```python
from build123d import *

# Parameters (mm, degrees)
F0_W     = 70
F0_H     = 60
F1_DEPTH = 2
F2_R     = 7
F3_W     = 64
F3_H     = 54
F4_DEPTH = 3
F5_R     = 5
F6_T     = -2


with BuildPart() as f1:
    # F0 (on Front) → F1 (new body)
    with BuildSketch(Plane.XZ):
        Rectangle(F0_W, F0_H)
    extrude(amount=F1_DEPTH)

    # F2
    f2_edges = [f1.edges().sort_by_distance(p)[0] for p in [
        (-35, -1, 30),
        (35, -1, 30),
        (35, -1, -30),
        (-35, -1, -30),
    ]]
    fillet(f2_edges, radius=F2_R)

    # F3 (on face) → F4 (join)
    with BuildSketch(Plane(origin=(0, 0, 0), x_dir=(-1, 0, 0), z_dir=(0, 1, 0))):
        Rectangle(F3_W, F3_H)
    extrude(amount=F4_DEPTH)

    # F5
    f5_edges = [f1.edges().sort_by_distance(p)[0] for p in [
        (32, 1.5, 27),
        (-32, 1.5, 27),
        (32, 1.5, -27),
        (-32, 1.5, -27),
    ]]
    fillet(f5_edges, radius=F5_R)

    # F6
    f6_openings = [f1.faces().sort_by_distance(p)[0] for p in [
        (0, 3, 0),
    ]]
    offset(amount=F6_T, openings=f6_openings, kind=Kind.INTERSECTION)


solid = f1.part
```
Verification items for the finished model (mm, model axes). A direction names the side the tool comes from. Give positions to 0.01 mm unless a question says otherwise; leave off trailing zeros. Order: outer loops, then holes, each group sorted by start corner. A loop starts at its lowest first (then second) coordinate and runs counter-clockwise, first axis right, second up. Notation, with made-up numbers: M 0,45 L 14,45 A8 ccw 14,50 Z; hole C 25.5,66 d7. An arc over 180 degrees is marked long. Answer in a Markdown table with one row per item. Add a question column.
Item 1: Mould release check, pull along Z, two halves, no side actions. Record for faces 5 (the cylindrical face through (-29.1, 1.52, 24.14)), 6 (the flat face through (35, -1, 0)), 7 (the flat face through (0, 1, -25)), 8 (the cylindrical face through (-33, -1, 27.9)): released by +Z, released by -Z, zero draft, split by the parting line, or undercut.
Item 2: Section check A-A, the plane y = 1.8. Enter the section's corners in (x, z).
Item 3: Section check B-B, the plane x = -1. Enter the section's corners in (y, z), and give its area (3 significant figures).
Item 4: Section check C-C, the plane z = 7.5. Enter the section's corners in (x, y).
Item 5: Scan lines: probe 1 along X at (y, z) = (0.6, 3); probe 2 along Z at (x, y) = (26, 0.9); probe 3 along Y at (x, z) = (8, 22). Record each from-to range of solid material in increasing order. Write a range as from..to.
Item 6: Tool access check on faces 1 (the flat face through (0, 1, 27)), 2 (the cylindrical face through (31, 2, 25)), 3 (the flat face through (-32, 1, 0)), 4 (the flat face through (30, 1, 0)). Record the directions out of +Z, -Z, +X, -X, +Y, -Y that give a thin tool (end or side, any length) a straight path to the whole face; none if there is none.
Item 7: Gauge pin test, flat ends, axial feed: pin 1 (18 mm diameter, centred on x = 7, z = 11.5, fed in from +Y); pin 2 (0.9 mm diameter, centred on y = 1.5, z = 10, fed in from +X); pin 3 (1 mm diameter, centred on x = 27, y = 1.5, fed in from -Z). Record the tip position at first contact, or that the pin passes through.
Filled sheet:
| question | item | result |
|---|---|---|
| 1 | face 5 | undercut |
| 1 | face 6 | zero draft |
| 1 | face 7 | undercut |
| 1 | face 8 | released by +Z |
| 2 | outline | M -32,-22 A5 ccw -27,-27 L 27,-27 A5 ccw 32,-22 L 32,22 A5 ccw 27,27 L -27,27 A5 ccw -32,22 Z; hole M -30,-22 A3 ccw -27,-25 L 27,-25 A3 ccw 30,-22 L 30,22 A3 ccw 27,25 L -27,25 A3 ccw -30,22 Z |
| 3 | outline | M -2,-30 L 0,-30 L 0,-27 L 3,-27 L 3,-25 L 0,-25 L 0,25 L 3,25 L 3,27 L 0,27 L 0,30 L -2,30 Z |
| 3 | area | 132 mm^2 |
| 4 | outline | M -35,-2 L 35,-2 L 35,0 L 32,0 L 32,3 L 30,3 L 30,0 L -30,0 L -30,3 L -32,3 L -32,0 L -35,0 Z |
| 5 | probe 1 | x = -32..-30, 30..32 |
| 5 | probe 2 | z = -27..-25, 25..27 |
| 5 | probe 3 | y = -2..0 |
| 6 | face 1 | +Z, +X, -X, +Y |
| 6 | face 2 | +Z, +X, +Y |
| 6 | face 3 | +Z, -Z, -X, +Y |
| 6 | face 4 | +Y |
| 7 | pin 1 | stops at y = 0 |
| 7 | pin 2 | stops at x = 32 |
| 7 | pin 3 | stops at z = -27 |
